Here's how the part is built. I have some questions about the finished solid (model axes, mm). A direction names the side the tool comes from. Give positions to 0.01 mm unless a question says otherwise; leave off trailing zeros. Loops run counter-clockwise (first coordinate to the right, second up) from the corner with the lowest first, then second, coordinate; pieces in that order, holes last.
Q1. I need wall thicknesses on probe 1 along Y at (x, z) = (26, -543); probe 2 along Z at (x, y) = (136, 49.5); probe 3 along Y at (x, z) = (136, -231). Which ranges of each line are inside material? Lowest first, please.
Q2. Suppose I cut it at B-B (z = -460.5). Count the separate pieces of the cut face and the enclosed holes in it, and give its area (3 significant figures).
Q3. Suppose I cut it at C-C (y = 674.5). List the corners of the cut face in (x, z) for me, and give its area (3 significant figures).
Q4. For faces 1 (the face through (76.2, 13, -301)), 2 (the face through (140, 0, -308)), 3 (the face through (127, 725, -584)), 4 (the face through (127, -25, -301)), 5 (the face through (140, -50.8, -301)), which set-ups out of +Z, -Z, +X, -X, +Y, -Y let a thin tool reach every point of the face, with its end or its side?
Q5. Suppose I cut it at D-D (x = 143). List the corners of the cut face in (y, z) for me.
Q6. Thinking about a two-plate mould opening in X: for faces 6 (the face through (152.4, 312, -574)), 7 (the face through (13, -50.8, -301)), 8 (the face through (64, 0, -301)), which applies, pulls with the +X half, pulls with the -X half, needs draft (parallel to the pull), parting line crosses it, or undercut?
Q7. Suppose I cut it at A-A (x = 41). List the corners of the cut face in (y, z) for me, and give its area (3 significant figures).
Q8. I'm going to push flat-ended pins straight in: P1, Ø7.5, axis at y = 414.5, z = -307.5, coming from the +X side; P2, Ø3, axis at y = 198.5, z = -187.5, coming from the +X side. Where does each tip first touch, or does it pass through?
```python
from build123d import *

# Parameters (mm, degrees)
F1_DEPTH = 609.6
F2_W     = 25.4
F2_H     = 50.8
F2_H_2   = 838.2
F3_DEPTH = 609.6
F4_W     = 838.2
F4_H     = 508
F5_DEPTH = 76.2


with BuildPart() as f1:
    # F0 (on Top) → F1 (new body)
    with BuildSketch(Plane.XY):
        Polygon((152.4, 838.2), (0, 838.2), (0, 419.1), (0, 0), (152.4, 0), (152.4, 25.4), (25.4, 25.4), (25.4, 203.2), (152.4, 203.2), (152.4, 215.9), (152.4, 228.6), (25.4, 228.6), (25.4, 406.4), (152.4, 406.4), (152.4, 419.1), (152.4, 431.8), (25.4, 431.8), (25.4, 609.6), (152.4, 609.6), (152.4, 622.3), (152.4, 635), (25.4, 635), (25.4, 812.8), (152.4, 812.8), align=None)
    extrude(amount=-F1_DEPTH)

    # F2 (on face) → F3 (join)
    with BuildSketch(Plane.XY):
        with Locations((12.7, 863.6)):
            Rectangle(F2_W, F2_H)
        with Locations((12.7, -25.4)):
            Rectangle(F2_W, F2_H)
        with Locations((139.7, 419.1)):
            Rectangle(F2_W, F2_H_2)
        with Locations((139.7, 863.6)):
            Rectangle(F2_W, F2_H)
        with Locations((139.7, -25.4)):
            Rectangle(F2_W, F2_H)
    extrude(amount=-F3_DEPTH)

    # F4 (on face) → F5 (cut)
    with BuildSketch(Plane.YZ.offset(152.4)):
        with Locations((419.1, -304.8)):
            Rectangle(F4_W, F4_H)
    extrude(amount=-F5_DEPTH, mode=Mode.SUBTRACT)


solid = f1.part
```
Solutions:
1. probe 1: y = 0 to 25.4, 203.2 to 228.6, 406.4 to 431.8, 609.6 to 635, 812.8 to 838.2
1. probe 2: z = -609.6 to -558.8, -50.8 to 0
1. probe 3: y = -50.8 to 0, 838.2 to 889
2. separate pieces: 3
2. enclosed holes: 0
2. area: 32,900 mm2
3. outline: (0, -609.6) - (25.4, -609.6) - (25.4, 0) - (0, 0) - close; (127, -609.6) - (152.4, -609.6) - (152.4, -558.8) - (127, -558.8) - close; (127, -50.8) - (152.4, -50.8) - (152.4, 0) - (127, 0) - close
3. area: 18,100 mm2
4. face 1: +X, +Y, -Y
4. face 2: +X
4. face 3: +Z, -Z
4. face 4: +Z, -Z, -Y
4. face 5: +Z, -Z, +X, -X, -Y
5. outline: (-50.8, -609.6) - (889, -609.6) - (889, 0) - (-50.8, 0) - close; hole (0, -558.8) - (838.2, -558.8) - (838.2, -50.8) - (0, -50.8) - close
6. face 6: pulls with the +X half
6. face 7: needs draft
6. face 8: undercut
7. outline: (0, -609.6) - (25.4, -609.6) - (25.4, 0) - (0, 0) - close; (203.2, -609.6) - (228.6, -609.6) - (228.6, 0) - (203.2, 0) - close; (406.4, -609.6) - (431.8, -609.6) - (431.8, 0) - (406.4, 0) - close; (609.6, -609.6) - (635, -609.6) - (635, 0) - (609.6, 0) - close; (812.8, -609.6) - (838.2, -609.6) - (838.2, 0) - (812.8, 0) - close
7. area: 77,400 mm2
8. P1: stops at x = 76.2
8. P2: stops at x = 25.4
